```python
from build123d import *

# Parameters (mm, degrees)
BOSS_EXTRUDE1_DEPTH = 10
SKETCH2_R           = 20.5
CUT_EXTRUDE1_DEPTH  = 5
SKETCH4_R           = 5
CUT_EXTRUDE3_DEPTH  = 148.732867027
SKETCH5_R           = 5
CUT_EXTRUDE4_DEPTH  = 5
SKETCH6_W           = 10
SKETCH6_H           = 40
CUT_EXTRUDE5_DEPTH  = 5


with BuildPart() as part:
    # Sketch1 → Boss-Extrude1 (new body)
    with BuildSketch(Plane(origin=(0, 0, 0), x_dir=(0, 0, -1), z_dir=(1, 0, 0))):
        Polygon((-75, 70), (-120, 70), (-120, 55), (-130, 55), (-130, 15), (-120, 15), (-120, 0), (-75, 0), (-75, 5), (-35, 5), (-35, 0), (-10, 0), (0, 0), (0, 15), (0, 55), (0, 70), (-10, 70), (-35, 70), (-35, 60), (-75, 60), align=None)
    extrude(amount=BOSS_EXTRUDE1_DEPTH)

    # Sketch2 → Cut-Extrude1 (cut)
    with BuildSketch(Plane(origin=(10, 0, 0), x_dir=(0, 0, -1), z_dir=(1, 0, 0))):
        with Locations((-88.52, 40)):
            Circle(SKETCH2_R)
    extrude(amount=-CUT_EXTRUDE1_DEPTH, mode=Mode.SUBTRACT)

    # Sketch4 → Cut-Extrude3 (cut, through all)
    with BuildSketch(Plane(origin=(5, 0, 0), x_dir=(0, 0, -1), z_dir=(1, 0, 0))):
        with Locations((-88.52, 40)):
            Circle(SKETCH4_R)
    extrude(amount=-CUT_EXTRUDE3_DEPTH, mode=Mode.SUBTRACT)

    # Sketch5 → Cut-Extrude4 (cut)
    with BuildSketch(Plane.ZY):
        with Locations((17.11, 26.509090973)):
            Circle(SKETCH5_R)
        with Locations((52.52, 33)):
            Circle(SKETCH5_R)
    extrude(amount=-CUT_EXTRUDE4_DEPTH, mode=Mode.SUBTRACT)

    # Sketch6 → Cut-Extrude5 (cut)
    with BuildSketch(Plane.ZY):
        with Locations((5, 35)):
            Rectangle(SKETCH6_W, SKETCH6_H)
    extrude(amount=-CUT_EXTRUDE5_DEPTH, mode=Mode.SUBTRACT)


solid = part.part
```
The listing builds one solid part. Answer for the finished solid, in the listing's coordinates (mm). A direction names the side the tool comes from. Coordinates: 2 decimals unless noted, no trailing zeros. Write each loop counter-clockwise with the first axis right and the second up, starting at its lowest first coordinate (ties: lowest second). Pieces come first, ordered by that corner, then holes. Notation, with made-up numbers: (42.5, 55.5) - (63.5, 55.5) arc R21 ccw to (63.5, 63.5) - close; hole circle Ø4 at (-38, -25.5). An arc over 180 degrees is marked (long way). Return JSON: item names as keys, results as strings. Group by question number.
1. Straight lines are drawn through the part: L1, parallel to Y at x = 7.4, z = 88.52; L2, parallel to Y at x = 2.2, z = 52.52; L3, parallel to Z at x = 6, y = 47. For each, find the intervals that lie inside material, in ascending order.
2. A cutting plane is placed at B-B, the plane z = 52.52. Determine the outline of the cut face in (x, y), plus the area to 3 significant figures.
3. A cutting plane is placed at D-D, the plane y = 50. Determine the outline of the cut face in (x, z), plus the area to 3 significant figures.
4. Determine the mould class of faces 4 (the flat face through (5, 3, 35)), 5 (the flat face through (2, 15, 5)), 6 (the flat face through (2, 35, 10)), 7 (the flat face through (5, 63, 120)) for opening direction Z: released by +Z, released by -Z, zero draft, split by the parting line, or undercut.
5. Which of the six approach directions +Z, -Z, +X, -X, +Y, -Y give full straight-line access (tool end or side, diameter ignored) to faces 1 (the flat face through (5, 35, 5)), 2 (the flat face through (5, 65, 35)), 3 (the flat face through (5, 27, 17))?
6. A cutting plane is placed at C-C, the plane x = 3. Determine the outline of the cut face in (y, z).
7. A cutting plane is placed at A-A, the plane y = 40. Determine the outline of the cut face in (x, z).
8. Given pin 1 (3 mm diameter, centred on x = 4.5, y = 16.5, fed in from -Z); pin 2 (3 mm diameter, centred on x = 6, y = 11, fed in from +Z); pin 3 (16 mm diameter, centred on y = 40, z = 88.52, fed in from +X); pin 4 (3 mm diameter, centred on x = 6, z = 61, fed in from +Y), each flat-ended and moving along its own axis, determine where each tip first touches the part or whether it passes through.
Ans:
{
 "1": {"L1": "0 to 19.5, 60.5 to 70", "L2": "5 to 28, 38 to 60", "L3": "0 to 69.25, 107.79 to 130"},
 "2": {"outline": "(0, 5) - (10, 5) - (10, 60) - (0, 60) - (0, 38) - (5, 38) - (5, 28) - (0, 28) - close", "area": "500 mm²"},
 "3": {"outline": "(0, 10) - (5, 10) - (5, 0) - (10, 0) - (10, 70.62) - (5, 70.62) - (5, 106.42) - (10, 106.42) - (10, 130) - (0, 130) - close", "area": "1,070 mm²"},
 "4": {"face 4": "undercut", "face 5": "zero draft", "face 6": "released by -Z", "face 7": "released by +Z"},
 "5": {"face 1": "-Z, -X", "face 2": "+X, -X, +Y", "face 3": "-X"},
 "6": {"outline": "(0, 0) - (15, 0) - (15, 10) - (55, 10) - (55, 0) - (70, 0) - (70, 35) - (60, 35) - (60, 75) - (70, 75) - (70, 120) - (55, 120) - (55, 130) - (15, 130) - (15, 120) - (0, 120) - (0, 75) - (5, 75) - (5, 35) - (0, 35) - close; hole circle Ø10 at (26.51, 17.11); hole circle Ø10 at (33, 52.52); hole circle Ø10 at (40, 88.52)"},
 "7": {"outline": "(0, 10) - (5, 10) - (5, 0) - (10, 0) - (10, 68.02) - (5, 68.02) - (5, 83.52) - (0, 83.52) - close; (0, 93.52) - (5, 93.52) - (5, 109.02) - (10, 109.02) - (10, 130) - (0, 130) - close"},
 "8": {"pin 1": "z = 0", "pin 2": "z = 120", "pin 3": "x = 5", "pin 4": "y = 60"}
}
